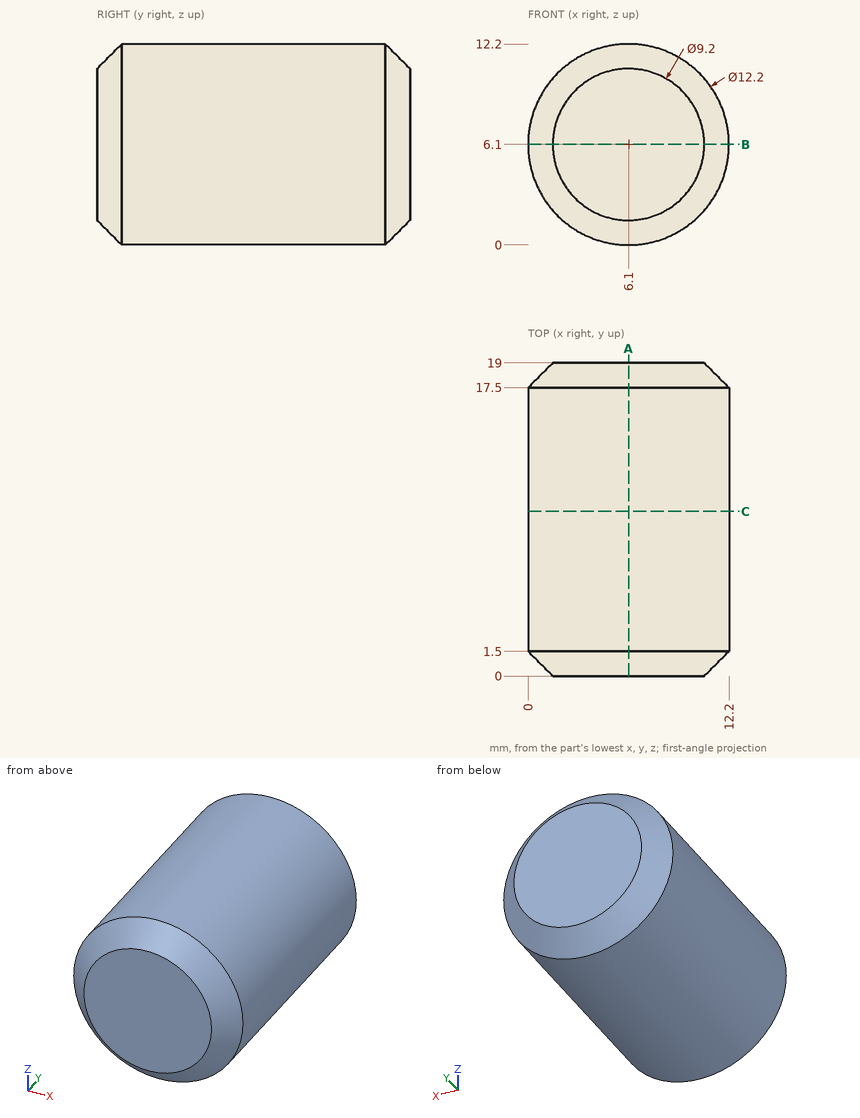
For this review, use the dimensioned drawing (mm, ordinates from the lowest corner) and the shaded views. Round coordinates to 2 decimals unless told otherwise and drop trailing zeros. Write each loop counter-clockwise with the first axis right and the second up, starting at its lowest first coordinate (ties: lowest second). Pieces come first, ordered by that corner, then holes. Notation, with made-up numbers: (-7, 71) -> (1, 71) arc R18 ccw to (1, 78) -> close; hole circle Ø5 at (-25, -32.5). An arc over 180 degrees is marked (long way). Use CSV: the item, a comma, the result in double quotes.
(1) Clearance check with flat-ended pins moving along their axes: P1, Ø3, axis at x = 3, y = 10, coming from the +Z side; P2, Ø1.5, axis at x = 1.5, z = 2, coming from the +Y side; P3, Ø4, axis at x = 3, y = 14, coming from the +Z side. State where each tip first meets the part, or that it passes through.
Computed values:
P1,"z = 11.99"
P2,"y = 18.19"
P3,"z = 12.1"
(2) To check wall thickness, follow L1, parallel to Y at x = 2.75, z = 2.25; L2, parallel to X at y = 10.75, z = 9; L3, parallel to Z at x = 5.75, y = 5. State the ranges of each line that lie inside material, in increasing order. Write a range as [from, to].
Computed values:
L1,"[0.5, 18.5]"
L2,"[0.73, 11.47]"
L3,"[0.01, 12.19]"
(3) Consider section B-B, the plane z = 6.1. Give the boundary of the cut face in (x, y), plus the area to 3 significant figures.
Computed values:
outline,"(0, 1.5) -> (1.5, 0) -> (10.7, 0) -> (12.2, 1.5) -> (12.2, 17.5) -> (10.7, 19) -> (1.5, 19) -> (0, 17.5) -> close"
area,"227 mm²"
(4) Consider section C-C, the plane y = 10. Give the boundary of the cut face in (x, z), plus the area to 3 significant figures.
Computed values:
outline,"circle Ø12.2 at (6.1, 6.1)"
area,"117 mm²"
(5) Consider section A-A, the plane x = 6.1. Give the boundary of the cut face in (y, z).
Computed values:
outline,"(0, 1.5) -> (1.5, 0) -> (17.5, 0) -> (19, 1.5) -> (19, 10.7) -> (17.5, 12.2) -> (1.5, 12.2) -> (0, 10.7) -> close"
